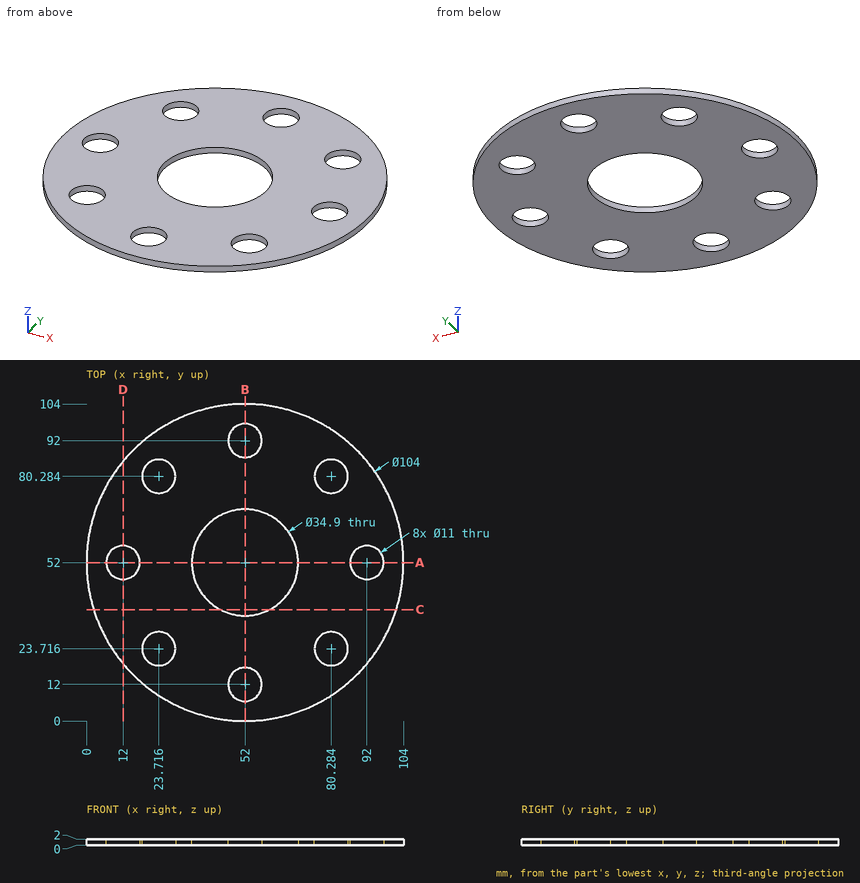
Part print with two shaded views. Sizes in mm from the minimum x, y, z corner. Give positions to 0.01 mm unless a question says otherwise; leave off trailing zeros. Order: outer loops, then holes, each group sorted by start corner. A loop starts at its lowest first (then second) coordinate and runs counter-clockwise, first axis right, second up.
(1) Saw through at D-D, the plane x = 12. Give the cut face in (y, z), then the cut area to 3 significant figures.
(2) Drill centre lines: L1, parallel to Y at x = 51, z = 0.8; L2, parallel to X at y = 81, z = 0.95; L3, parallel to X at y = 50.5, z = 0.3 (1 decimal). Where is each one in solid material? Low to high.
(3) Saw through at C-C, the plane y = 36.5. Give the cut face in (x, z).
(4) Saw through at A-A, the plane y = 52. Give the cut face in (x, z).
(5) Flat gauge pins, fed straight in: pin 1 (1 mm diameter, centred on x = 80.5, z = 1, fed in from +Y); pin 2 (1 mm diameter, centred on y = 45.5, z = 1, fed in from -X); pin 3 (17.5 mm diameter, centred on x = 12, y = 52, fed in from +Z); pin 4 (9 mm diameter, centred on x = 23.72, y = 23.72, fed in from -Z). Where does each tip first touch, or does it go through?
Results found:
1. outline: (18.77, 0) - (46.5, 0) - (46.5, 2) - (18.77, 2) - close; (57.5, 0) - (85.23, 0) - (85.23, 2) - (57.5, 2) - close
1. area: 111 mm2
2. L1: y = 0.01 to 6.59, 17.41 to 34.58, 69.42 to 86.59, 97.41 to 103.99
2. L2: x = 8.84 to 18.26, 29.17 to 74.83, 85.74 to 95.16
2. L3: x = 0 to 6.7, 17.3 to 34.6, 69.4 to 86.7, 97.3 to 104
3. outline: (2.36, 0) - (43.98, 0) - (43.98, 2) - (2.36, 2) - close; (60.02, 0) - (101.64, 0) - (101.64, 2) - (60.02, 2) - close
4. outline: (0, 0) - (6.5, 0) - (6.5, 2) - (0, 2) - close; (17.5, 0) - (34.55, 0) - (34.55, 2) - (17.5, 2) - close; (69.45, 0) - (86.5, 0) - (86.5, 2) - (69.45, 2) - close; (97.5, 0) - (104, 0) - (104, 2) - (97.5, 2) - close
5. pin 1: stops at y = 95.82
5. pin 2: stops at x = 0.35
5. pin 3: stops at z = 2
5. pin 4: passes through
